```python
from build123d import *

# Parameters (mm, degrees)
CROQUIS2_R              = 1.52
CROQUIS2_R_2            = 2.4
CROQUIS2_R_3            = 1.59
CROQUIS2_R_4            = 2
SALIENTE_EXTRUIR1_DEPTH = 2


with BuildPart() as part:
    # Croquis2 → Saliente-Extruir1 (new body)
    with BuildSketch(Plane(origin=(0, 0, 0), x_dir=(1, 0, 0), z_dir=(0, 1, 0))):
        with BuildLine():
            ThreePointArc((-15.6443026, -5.332651407), (-16.282242792, -8.847169319), (-18.114669831, -11.913276785))
            Line((-18.114669831, -11.913276785), (-25.665833323, -20.55341124))
            ThreePointArc((-25.665833323, -20.55341124), (-26.522572581, -23.091497469), (-25.333680736, -25.492001591))
            Line((-25.333680736, -25.492001591), (-21.870049663, -28.519089265))
            Line((-21.870049663, -28.519089265), (-18.053864835, -31.854296107))
            ThreePointArc((-18.053864835, -31.854296107), (-16.559946136, -32.720000224), (-14.85, -32.95941808))
            ThreePointArc((-14.85, -32.95941808), (-11.500177955, -29.398955686), (-15.258060002, -26.272212538))
            Line((-15.258060002, -26.272212538), (-9.898337732, -20.139552173))
            ThreePointArc((-9.898337732, -20.139552173), (-6.503541491, -17.615062127), (-2.368704963, -16.720177551))
            Line((-2.368704963, -16.720177551), (2.368704963, -16.720177551))
            ThreePointArc((2.368704963, -16.720177551), (6.503541491, -17.615062127), (9.898337732, -20.139552173))
            Line((9.898337732, -20.139552173), (15.258060002, -26.272212538))
            ThreePointArc((15.258060002, -26.272212538), (11.500177955, -29.398955686), (14.85, -32.95941808))
            ThreePointArc((14.85, -32.95941808), (16.559946136, -32.720000224), (18.053864835, -31.854296107))
            Line((18.053864835, -31.854296107), (21.870049663, -28.519089265))
            Line((21.870049663, -28.519089265), (25.333680736, -25.492001591))
            ThreePointArc((25.333680736, -25.492001591), (26.522572581, -23.091497469), (25.665833323, -20.55341124))
            Line((25.665833323, -20.55341124), (18.114669831, -11.913276785))
            ThreePointArc((18.114669831, -11.913276785), (16.282242792, -8.847169319), (15.6443026, -5.332651407))
            Line((15.6443026, -5.332651407), (15.6443026, 5.332651407))
            ThreePointArc((15.6443026, 5.332651407), (16.282242792, 8.847169319), (18.114669831, 11.913276785))
            Line((18.114669831, 11.913276785), (25.665833323, 20.55341124))
            ThreePointArc((25.665833323, 20.55341124), (26.522572581, 23.091497469), (25.333680736, 25.492001591))
            Line((25.333680736, 25.492001591), (21.870049663, 28.519089265))
            Line((21.870049663, 28.519089265), (18.053864835, 31.854296107))
            ThreePointArc((18.053864835, 31.854296107), (16.559946136, 32.720000224), (14.85, 32.95941808))
            ThreePointArc((14.85, 32.95941808), (11.500177955, 29.398955686), (15.258060002, 26.272212538))
            Line((15.258060002, 26.272212538), (9.898337732, 20.139552173))
            ThreePointArc((9.898337732, 20.139552173), (6.503541491, 17.615062127), (2.368704963, 16.720177551))
            Line((2.368704963, 16.720177551), (-2.368704963, 16.720177551))
            ThreePointArc((-2.368704963, 16.720177551), (-6.503541491, 17.615062127), (-9.898337732, 20.139552173))
            Line((-9.898337732, 20.139552173), (-15.258060002, 26.272212538))
            ThreePointArc((-15.258060002, 26.272212538), (-11.500177955, 29.398955686), (-14.85, 32.95941808))
            ThreePointArc((-14.85, 32.95941808), (-16.559946136, 32.720000224), (-18.053864835, 31.854296107))
            Line((-18.053864835, 31.854296107), (-21.870049663, 28.519089265))
            Line((-21.870049663, 28.519089265), (-25.333680736, 25.492001591))
            ThreePointArc((-25.333680736, 25.492001591), (-26.522572581, 23.091497469), (-25.665833323, 20.55341124))
            Line((-25.665833323, 20.55341124), (-18.114669831, 11.913276785))
            ThreePointArc((-18.114669831, 11.913276785), (-16.282242792, 8.847169319), (-15.6443026, 5.332651407))
            Line((-15.6443026, 5.332651407), (-15.6443026, -5.332651407))
        make_face()
        with Locations(Location((-14.85, -29.603365193, 0), (0, 0, 270))):
            Circle(CROQUIS2_R, mode=Mode.SUBTRACT)
        with Locations(Location((-20.768636021, -24.348641057, 0), (0, 0, 270))):
            Circle(CROQUIS2_R_2, mode=Mode.SUBTRACT)
        with Locations(Location((-15.030603638, -15.334854811, 0), (0, 0, 270))):
            Circle(CROQUIS2_R_3, mode=Mode.SUBTRACT)
        with Locations(Location((-0.05, -12.497128708, 0), (0, 0, 270))):
            Circle(CROQUIS2_R_4, mode=Mode.SUBTRACT)
        with BuildLine():
            Line((-3.074423593, -5.999581964), (-5.873559772, -10.915994174))
            ThreePointArc((-5.873559772, -10.915994174), (-7.324662306, -11.905756202), (-8.997091839, -11.368814033))
            Line((-8.997091839, -11.368814033), (-10.997834751, -9.446969084))
            ThreePointArc((-10.997834751, -9.446969084), (-11.601593103, -7.79748332), (-10.670982222, -6.30775488))
            Line((-10.670982222, -6.30775488), (-5.87110313, -3.313187619))
            ThreePointArc((-5.87110313, -3.313187619), (-3.426979279, -3.567667883), (-3.074423593, -5.999581964))
        make_face(mode=Mode.SUBTRACT)
        with Locations(Location((14.85, -29.603365193, 0), (0, 0, 270))):
            Circle(CROQUIS2_R, mode=Mode.SUBTRACT)
        with Locations(Location((21.231326929, -24.292854014, 0), (0, 0, 270))):
            Circle(CROQUIS2_R_2, mode=Mode.SUBTRACT)
        with BuildLine():
            Line((10.997834751, -9.446969084), (8.997091839, -11.368814033))
            ThreePointArc((8.997091839, -11.368814033), (7.324662306, -11.905756202), (5.873559772, -10.915994174))
            Line((5.873559772, -10.915994174), (3.074423593, -5.999581964))
            ThreePointArc((3.074423593, -5.999581964), (3.426979279, -3.567667883), (5.87110313, -3.313187619))
            Line((5.87110313, -3.313187619), (10.670982222, -6.30775488))
            ThreePointArc((10.670982222, -6.30775488), (11.601593103, -7.79748332), (10.997834751, -9.446969084))
        make_face(mode=Mode.SUBTRACT)
        with Locations(Location((15.469369457, -15.294342791, 0), (0, 0, 270))):
            Circle(CROQUIS2_R_3, mode=Mode.SUBTRACT)
        with Locations(Location((-15.071115657, 15.165118284, 0), (0, 0, 270))):
            Circle(CROQUIS2_R_3, mode=Mode.SUBTRACT)
        with BuildLine():
            Line((-10.997834751, 9.446969084), (-8.997091839, 11.368814033))
            ThreePointArc((-8.997091839, 11.368814033), (-7.324662306, 11.905756202), (-5.873559772, 10.915994174))
            Line((-5.873559772, 10.915994174), (-3.074423593, 5.999581964))
            ThreePointArc((-3.074423593, 5.999581964), (-3.426979279, 3.567667883), (-5.87110313, 3.313187619))
            Line((-5.87110313, 3.313187619), (-10.670982222, 6.30775488))
            ThreePointArc((-10.670982222, 6.30775488), (-11.601593103, 7.79748332), (-10.997834751, 9.446969084))
        make_face(mode=Mode.SUBTRACT)
        with Locations(Location((-0.05, 12.497128708, 0), (0, 0, 270))):
            Circle(CROQUIS2_R_4, mode=Mode.SUBTRACT)
        with Locations(Location((-20.833073129, 24.163629506, 0), (0, 0, 270))):
            Circle(CROQUIS2_R_2, mode=Mode.SUBTRACT)
        with Locations(Location((-14.85, 29.603365193, 0), (0, 0, 270))):
            Circle(CROQUIS2_R, mode=Mode.SUBTRACT)
        with BuildLine():
            Line((3.074423593, 5.999581964), (5.873559772, 10.915994174))
            ThreePointArc((5.873559772, 10.915994174), (7.324662306, 11.905756202), (8.997091839, 11.368814033))
            Line((8.997091839, 11.368814033), (10.997834751, 9.446969084))
            ThreePointArc((10.997834751, 9.446969084), (11.601593103, 7.79748332), (10.670982222, 6.30775488))
            Line((10.670982222, 6.30775488), (5.87110313, 3.313187619))
            ThreePointArc((5.87110313, 3.313187619), (3.426979279, 3.567667883), (3.074423593, 5.999581964))
        make_face(mode=Mode.SUBTRACT)
        with Locations(Location((15.428857437, 15.205630304, 0), (0, 0, 270))):
            Circle(CROQUIS2_R_3, mode=Mode.SUBTRACT)
        with Locations(Location((21.166889821, 24.21941655, 0), (0, 0, 270))):
            Circle(CROQUIS2_R_2, mode=Mode.SUBTRACT)
        with Locations(Location((14.85, 29.603365193, 0), (0, 0, 270))):
            Circle(CROQUIS2_R, mode=Mode.SUBTRACT)
    extrude(amount=SALIENTE_EXTRUIR1_DEPTH)


solid = part.part
```
Geometry: final body of the model. Coordinates: model frame, mm. A direction names the side the tool comes from. Round coordinates to 2 decimals unless told otherwise and drop trailing zeros. Write each loop counter-clockwise with the first axis right and the second up, starting at its lowest first coordinate (ties: lowest second). Pieces come first, ordered by that corner, then holes. Notation, with made-up numbers: (27, -10) -> (52, -10) arc R6 cw to (52, -1) -> close; hole circle Ø3 at (-9.5, -29.75). An arc over 180 degrees is marked (long way). Return JSON: item names as keys, results as strings.
Q1. Set-up query: faces 1 (the flat face through (8.24, 0.99, 4.79)), 2 (the cylindrical face through (-16.265, 0.986, 8.8)), 3 (the cylindrical face through (6.45, 0.99, 17.59)). Return all of +Z, -Z, +X, -X, +Y, -Y with unobstructed straight access to the full face (end or side cutting, diameter ignored); none if empty.
From the geometry:
{"face 1": "+Y, -Y", "face 2": "-X, +Y, -Y", "face 3": "+Z, +Y, -Y"}
Q2. Ray query, line 1 (Z direction, x = 0, y = 0.95); line 2 (Z direction, x = 3, y = 1.2); line 3 (X direction, y = 1, z = -8). Return the intervals inside material, ascending.
From the geometry:
{"line 1": "-16.72 to -14.5, -10.5 to 10.5, 14.5 to 16.72", "line 2": "-16.74 to -5.86, -4.16 to 4.16, 5.86 to 16.74", "line 3": "-16.01 to -11.61, -4.21 to 4.21, 11.61 to 16.01"}
Q3. First-contact query: pin 1 Ø3 at (x, z) = (21.17, -24.22) entering from +Y; pin 2 Ø1 at (y, z) = (0.5, 0) entering from +X; pin 3 Ø1 at (y, z) = (0.5, -1) entering from -X. Flat tips, straight axial feed; report the tip coordinate or a pass-through.
From the geometry:
{"pin 1": "through", "pin 2": "x = 15.64", "pin 3": "x = -15.64"}
Q4. Section A-A on x = -0.05. Return the cut outline in (y, z).
From the geometry:
{"outline": "(0, -16.72) -> (2, -16.72) -> (2, -14.5) -> (0, -14.5) -> close; (0, -10.5) -> (2, -10.5) -> (2, 10.5) -> (0, 10.5) -> close; (0, 14.5) -> (2, 14.5) -> (2, 16.72) -> (0, 16.72) -> close"}
Q5. Mould query, pull axis Z, two halves, no side actions, for faces 4 (the cylindrical face through (-11.6, 1, -7.8)), 5 (the flat face through (-12.616, 0.986, 23.249)), 6 (the flat face through (0, 0, 0)), 7 (the cylindrical face through (-16.537, 0.986, -32.728)). Classes: +Z half, -Z half, draft (parallel to the pull), parting line (faces both ways), or undercut.
From the geometry:
{"face 4": "undercut", "face 5": "undercut", "face 6": "draft", "face 7": "-Z half"}
Q6. Section C-C on z = -1. Return the cut outline in (x, y).
From the geometry:
{"outline": "(-15.64, 0) -> (15.64, 0) -> (15.64, 2) -> (-15.64, 2) -> close"}
Q7. Section D-D on x = -7. Return the cut outline in (y, z), and give its area (3 significant figures).
From the geometry:
{"outline": "(0, -17.86) -> (2, -17.86) -> (2, -11.83) -> (0, -11.83) -> close; (0, -4.02) -> (2, -4.02) -> (2, 4.02) -> (0, 4.02) -> close; (0, 11.83) -> (2, 11.83) -> (2, 17.86) -> (0, 17.86) -> close", "area": "40.2 mm2"}
Q8. Section B-B on z = -23. Return the cut outline in (x, y).
From the geometry:
{"outline": "(-26.53, 0) -> (-22.93, 0) -> (-22.93, 2) -> (-26.53, 2) -> close; (-18.73, 0) -> (-12.4, 0) -> (-12.4, 2) -> (-18.73, 2) -> close; (12.4, 0) -> (19.1, 0) -> (19.1, 2) -> (12.4, 2) -> close; (23.23, 0) -> (26.53, 0) -> (26.53, 2) -> (23.23, 2) -> close"}
